from build123d import *

# Parameters (mm, degrees)
SKETCH1_R           = 2.15
BOSS_EXTRUDE1_DEPTH = 10
SKETCH3_W           = 75
SKETCH3_H           = 3
CUT_EXTRUDE1_DEPTH  = 4


with BuildPart() as part:
    # Sketch1 → Boss-Extrude1 (new body)
    with BuildSketch(Plane.XY):
        Polygon((21, 5), (37.5, 5), (37.5, -20), (-37.5, -20), (-37.5, 5), (-21, 5), (-21, -10), (21, -10), align=None)
        with Locations((-30.5, 0)):
            Circle(SKETCH1_R, mode=Mode.SUBTRACT)
        with Locations((-30.5, -12)):
            Circle(SKETCH1_R, mode=Mode.SUBTRACT)
        with Locations((30.5, 0)):
            Circle(SKETCH1_R, mode=Mode.SUBTRACT)
        with Locations((30.5, -12)):
            Circle(SKETCH1_R, mode=Mode.SUBTRACT)
    extrude(amount=BOSS_EXTRUDE1_DEPTH)

    # Sketch3 → Cut-Extrude1 (cut)
    with BuildSketch(Plane(origin=(0, 0, 0), x_dir=(-1, 0, 0), z_dir=(0, 0, -1))):
        with Locations((0, -18.5)):
            Rectangle(SKETCH3_W, SKETCH3_H)
    extrude(amount=-CUT_EXTRUDE1_DEPTH, mode=Mode.SUBTRACT)


solid = part.part
Input: part model. Units: mm. Frame: model coordinates. A direction names the side the tool comes from. Coordinates: 2 decimals unless noted, no trailing zeros. Loops run counter-clockwise (first coordinate to the right, second up) from the corner with the lowest first, then second, coordinate; pieces in that order, holes last.
(1) Section A-A on y = -7.75. Return the cut outline in (x, z).
(2) First-contact query: pin 1 Ø3 at (x, z) = (-5.5, 5.5) entering from +Y; pin 2 Ø2 at (x, z) = (-15, 1) entering from -Y. Flat tips, straight axial feed; report the tip coordinate or a pass-through.
(3) Section C-C on y = -12. Return the cut outline in (x, z), then the cut area to 3 significant figures.
(4) Set-up query: faces 1 (the face through (0, -10, 5)), 2 (the face through (-29, 5, 5)), 3 (the face through (1, -18, 4)). Return all of +Z, -Z, +X, -X, +Y, -Y with unobstructed straight access to the full face (end or side cutting, diameter ignored); none if empty.
(5) Pull-direction query (Y, two-part tool) for faces 4 (the face through (21, -3, 5)), 5 (the face through (-28.45, 0.65, 4.93)), 6 (the face through (1, -17, 2)); classes: released by +Y, released by -Y, zero draft, split by the parting line, or undercut.
(6) Section B-B on x = 30.5. Return the cut outline in (y, z).
(7) Material intervals for probe 1 along X at (y, z) = (-0.25, 5.25); probe 2 along Y at (x, z) = (-30.5, 3.5); probe 3 along Y at (x, z) = (30.5, 4.5), sorted ascending.
(8) Section D-D on z = 3.25. Return the cut outline in (x, y).
Data:
1. outline: (-37.5, 0) - (-21, 0) - (-21, 10) - (-37.5, 10) - close; (21, 0) - (37.5, 0) - (37.5, 10) - (21, 10) - close
2. pin 1: stops at y = -10
2. pin 2: stops at y = -17
3. outline: (-37.5, 0) - (-32.65, 0) - (-32.65, 10) - (-37.5, 10) - close; (-28.35, 0) - (28.35, 0) - (28.35, 10) - (-28.35, 10) - close; (32.65, 0) - (37.5, 0) - (37.5, 10) - (32.65, 10) - close
3. area: 664 mm2
4. face 1: +Z, -Z, +Y
4. face 2: +Z, -Z, +X, -X, +Y
4. face 3: -Z, +X, -X, -Y
5. face 4: zero draft
5. face 5: undercut
5. face 6: released by -Y
6. outline: (-20, 4) - (-17, 4) - (-17, 0) - (-14.15, 0) - (-14.15, 10) - (-20, 10) - close; (-9.85, 0) - (-2.15, 0) - (-2.15, 10) - (-9.85, 10) - close; (2.15, 0) - (5, 0) - (5, 10) - (2.15, 10) - close
7. probe 1: x = -37.5 to -32.64, -28.36 to -21, 21 to 28.36, 32.64 to 37.5
7. probe 2: y = -17 to -14.15, -9.85 to -2.15, 2.15 to 5
7. probe 3: y = -20 to -14.15, -9.85 to -2.15, 2.15 to 5
8. outline: (-37.5, -17) - (37.5, -17) - (37.5, 5) - (21, 5) - (21, -10) - (-21, -10) - (-21, 5) - (-37.5, 5) - close; hole circle Ø4.3 at (-30.5, -12); hole circle Ø4.3 at (-30.5, 0); hole circle Ø4.3 at (30.5, -12); hole circle Ø4.3 at (30.5, 0)
